```python
from build123d import *

# Parameters (mm, degrees)
SKETCH1_W                   = 152.4
SKETCH1_H                   = 101.6
BOSS_EXTRUDE1_DEPTH         = 6.35
F_1_4_0_25_DIAMETER_HOLE1_D = 6.35
LPATTERN1_COUNT             = 2
LPATTERN1_PITCH             = 76.2
LPATTERN1_COUNT_DIR2        = 2
LPATTERN1_PITCH_DIR2        = 127
FILLET1_R                   = 6.35


with BuildPart() as part:
    # Sketch1 → Boss-Extrude1 (new body)
    with BuildSketch(Plane.ZY.offset(323.85)):
        with Locations((-342.9, 69.85)):
            Rectangle(SKETCH1_W, SKETCH1_H)
    extrude(amount=BOSS_EXTRUDE1_DEPTH)

    # 1/4 (0.25) Diameter Hole1 (through all)
    with Locations(Plane.ZY.offset(330.2)):
        with Locations((-406.4, 31.75)):
            f_1_4_0_25_diameter_hole1 = Hole(F_1_4_0_25_DIAMETER_HOLE1_D / 2)

    # LPattern1: 1_4 _0.25_ Diameter Hole1 2 × 2
    with Locations(*[(0, i * LPATTERN1_PITCH, j * LPATTERN1_PITCH_DIR2) for i in range(LPATTERN1_COUNT) for j in range(LPATTERN1_COUNT_DIR2) if (i, j) != (0, 0)]):
        add(f_1_4_0_25_diameter_hole1, mode=Mode.SUBTRACT)

    # Fillet1
    fillet1_edges = [part.edges().sort_by_distance(p)[0] for p in [
        (-327.025, 120.65, -419.1),
        (-327.025, 120.65, -266.7),
        (-327.025, 19.05, -266.7),
        (-327.025, 19.05, -419.1),
    ]]
    fillet(fillet1_edges, radius=FILLET1_R)


solid = part.part
```
Geometry check sheet. Reference: the model listing, model coordinates, mm. Coordinates: 2 decimals unless noted, no trailing zeros. Write each loop counter-clockwise with the first axis right and the second up, starting at its lowest first coordinate (ties: lowest second). Pieces come first, ordered by that corner, then holes. Notation, with made-up numbers: M 31,85.5 L 86,85.5 A25 ccw 86,113.5 Z; hole C 2,-35 d4. An arc over 180 degrees is marked long. One line per item, written item: value. Start each with the question number.
(1) Scan lines: line 1 along Y through (x, z) = (-327.75, -406.4) (3 decimals); line 2 along Z through (x, y) = (-325.5, 115); line 3 along Z through (x, y) = (-327, 116.5). Record each from-to range of solid material in increasing order. Write a range as [from, to].
(2) Sectioned sample at A-A, the plane y = 107.95. Enter the section's corners in (x, z) (3 decimals), and give its area (3 significant figures).
(3) Release check for a two-part mould opening along Y. For faces 1 (the face through (-327, 69, -419.1)), 2 (the face through (-327.07, 118.74, -417.29)), 3 (the face through (-326.98, 108.09, -403.23)), 4 (the face through (-327.07, 20.86, -268.61)) record: released by +Y, released by -Y, zero draft, split by the parting line, or undercut.
(4) Sectioned sample at B-B, the plane z = -406.4. Enter the section's corners in (x, y) (3 decimals).
(5) Depth check by flat-ended pin: pin 1 (5 mm diameter, centred on y = 107.95, z = -406.4, fed in from +X). Enter the tip coordinate at first touch or a pass-through.
Filled sheet:
1. line 1: [19.05, 28.575], [34.925, 104.775], [111.125, 120.65]
1. line 2: [-419.06, -266.74]
1. line 3: [-418.71, -267.09]
2. outline: M -330.2,-419.1 L -323.85,-419.1 L -323.85,-409.575 L -330.2,-409.575 Z; M -330.2,-403.225 L -323.85,-403.225 L -323.85,-282.575 L -330.2,-282.575 Z; M -330.2,-276.225 L -323.85,-276.225 L -323.85,-266.7 L -330.2,-266.7 Z
2. area: 887 mm²
3. face 1: zero draft
3. face 2: released by +Y
3. face 3: undercut
3. face 4: released by -Y
4. outline: M -330.2,19.05 L -323.85,19.05 L -323.85,28.575 L -330.2,28.575 Z; M -330.2,34.925 L -323.85,34.925 L -323.85,104.775 L -330.2,104.775 Z; M -330.2,111.125 L -323.85,111.125 L -323.85,120.65 L -330.2,120.65 Z
5. pin 1: through
